```python
from build123d import *

# Parameters (mm, degrees)
SKETCH1_W     = 3.5
SKETCH1_H     = 4
CHAMFER1_SIZE = 0.1


with BuildPart() as part:
    # Sketch1 → Revolve1 (revolve)
    with BuildSketch(Plane(origin=(0, 0, 0), x_dir=(0, 0, -1), z_dir=(1, 0, 0))):
        with Locations((3.25, 0)):
            Rectangle(SKETCH1_W, SKETCH1_H)
    revolve(axis=Axis((0, 2, 0), (0, -1, 0)))

    # Sketch3 → Cut-Revolve2 (revolve, cut)
    with BuildSketch(Plane(origin=(0, 0, 0), x_dir=(0, 0, -1), z_dir=(1, 0, 0))):
        Polygon((3.8, 1.8), (4, 1.6), (4, 2), (2.25, 2), (2.25, 1.6), (2.45, 1.8), align=None)
    cut_revolve2 = revolve(axis=Axis((0, 2, 0), (0, -1, 0)), mode=Mode.SUBTRACT)

    # Mirror1: Cut-Revolve2 across plane
    add(cut_revolve2.mirror(Plane.ZX), mode=Mode.SUBTRACT)

    # Chamfer1
    chamfer1_edges = [part.edges().sort_by_distance(p)[0] for p in [
        (0, 2, 4),
        (0, 2, 2.25),
        (0, -2, 4),
        (0, -2, 2.25),
        (0, 2, 5),
        (0, -2, 5),
        (0, -2, 1.5),
        (0, 2, 1.5),
    ]]
    chamfer(chamfer1_edges, length=CHAMFER1_SIZE)


solid = part.part
```
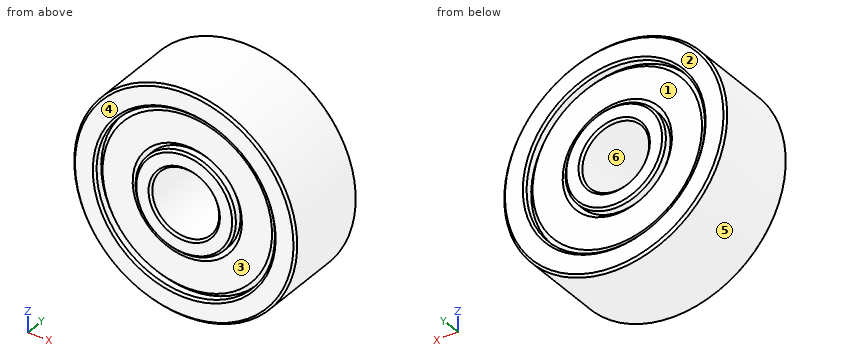
Source: CAD feature listing. Evaluate the final solid. Frame: model axes, mm. Face numbers are marked on the shaded views. A direction names the side the tool comes from. Coordinates: 2 decimals unless noted, no trailing zeros. Loops run counter-clockwise (first coordinate to the right, second up) from the corner with the lowest first, then second, coordinate; pieces in that order, holes last. Notation, with made-up numbers: M -8,12 L 20,12 A29 cw 20,38 Z; hole C -15.5,-11.5 d9. An arc over 180 degrees is marked long. Put each result on its own line as item: value. Start each with the question number.
1) Ray query, L1, parallel to X at y = 1.85, z = 0; L2, parallel to X at y = 1, z = 0; L3, parallel to X at y = -0.9, z = -3. Return the intervals inside material, ascending. Write a range as from..to.
2) Reachability of the marked faces 1 and 2 from +Z, -Z, +X, -X, +Y, -Y: full face, straight path, thin tool, end or side. Return the list, or none.
3) Cut plane A-A on y = 1.2. Return the cut outline in (x, z).
4) Pull-direction query (X, two-part tool) for the marked faces 3, 4, 5 and 6; classes: pulls with the +X half, pulls with the -X half, needs draft (parallel to the pull), parting line crosses it, or undercut.
The answers:
1. L1: x = -5..-4, -2.25..-1.5, 1.5..2.25, 4..5
1. L2: x = -5..-1.5, 1.5..5
1. L3: x = -4..4
2. face 1: +Y
2. face 2: +Z, -Z, +X, -X, +Y
3. outline: C 0,0 d10; hole C 0,0 d3
4. face 3: undercut
4. face 4: needs draft
4. face 5: parting line crosses it
4. face 6: undercut
